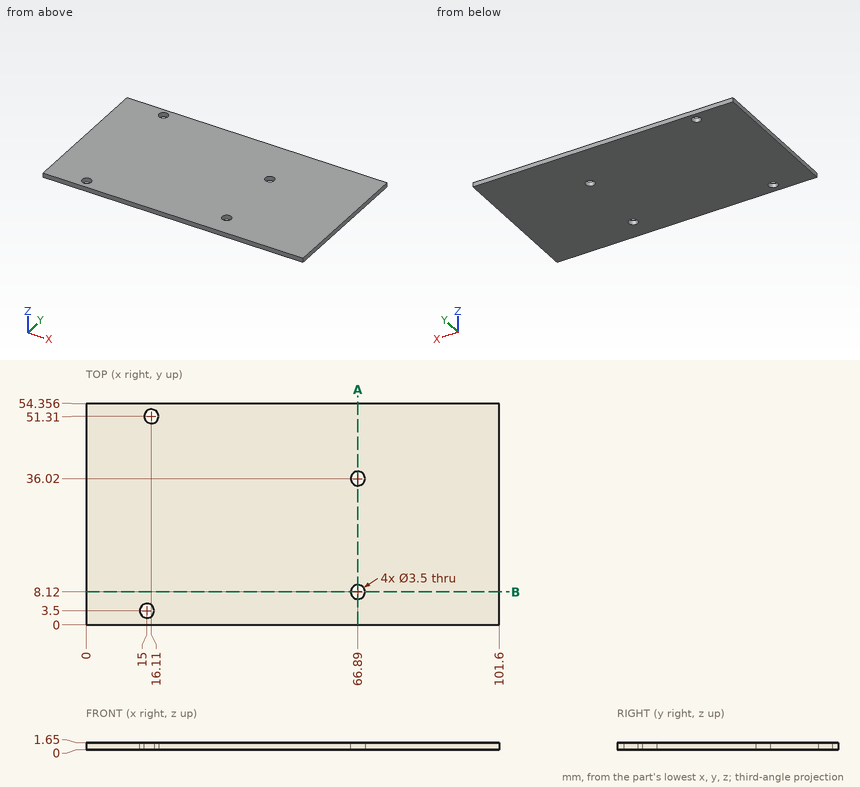
Job drawing, mm, ordinate dimensions from the low corner. One solid piece. Round coordinates to 2 decimals unless told otherwise and drop trailing zeros. Write each loop counter-clockwise with the first axis right and the second up, starting at its lowest first coordinate (ties: lowest second). Pieces come first, ordered by that corner, then holes. Notation, with made-up numbers: (-19.75, 47) -> (27.25, 47) arc R9 cw to (27.25, 57) -> close; hole circle Ø11 at (31, 10). An arc over 180 degrees is marked (long way). Answer as a JSON object with one key per item and string values.
(1) Band-saw the part on B-B, the plane y = 8.12. List the corners of the cut face in (x, z).
Reported:
{"outline": "(0, 0) -> (65.14, 0) -> (65.14, 1.65) -> (0, 1.65) -> close; (68.64, 0) -> (101.6, 0) -> (101.6, 1.65) -> (68.64, 1.65) -> close"}
(2) Probe probe 1 along X at (y, z) = (8, 0.2); probe 2 along Y at (x, z) = (15, 1.25); probe 3 along X at (y, z) = (35, 0.75). List the from-to ranges inside material, lowest first. Write a range as [from, to].
Reported:
{"probe 1": "x = [0, 65.14], [68.64, 101.6]", "probe 2": "y = [0, 1.75], [5.25, 49.96], [52.66, 54.36]", "probe 3": "x = [0, 65.47], [68.31, 101.6]"}
(3) Band-saw the part on A-A, the plane x = 66.89. List the corners of the cut face in (y, z), then the cut area to 3 significant figures.
Reported:
{"outline": "(0, 0) -> (6.37, 0) -> (6.37, 1.65) -> (0, 1.65) -> close; (9.87, 0) -> (34.27, 0) -> (34.27, 1.65) -> (9.87, 1.65) -> close; (37.77, 0) -> (54.36, 0) -> (54.36, 1.65) -> (37.77, 1.65) -> close", "area": "78.1 mm^2"}
